Check sheet for the modelled part. Datum: model origin and axes. Units: mm. Round coordinates to 2 decimals unless told otherwise and drop trailing zeros. Order: outer loops, then holes, each group sorted by start corner. A loop starts at its lowest first (then second) coordinate and runs counter-clockwise, first axis right, second up. Notation, with made-up numbers: M -18.5,89 L 9.5,89 A18 cw 9.5,115 Z; hole C 80,89.5 d10. An arc over 180 degrees is marked long. One line per item, written item: value. Start each with the question number.
(1) Thickness scan on L1, parallel to X at y = 5, z = -61.5; L2, parallel to X at y = 4, z = -65 (1 decimal); L3, parallel to Z at x = 895.35, y = 6. Record the ranges inside material, lowest first.
(2) Cross-section at A-A, the plane z = -52. Enter the section's corners in (x, y) (3 decimals), and give its area (3 significant figures).
(3) Cross-section at C-C, the plane y = 5. Count the separate pieces of the cut face and the enclosed holes in it, and give its area (3 significant figures).
(4) Depth check by flat-ended pin: pin 1 Ø5 at (x, y) = (202.5, 8) entering from -Z. Enter the tip coordinate at first touch or a pass-through.
(5) Cross-section at D-D, the plane x = 307. Enter the section's corners in (y, z) (3 decimals).
(6) Cross-section at B-B, the plane x = 756. Enter the section's corners in (y, z) (3 decimals).
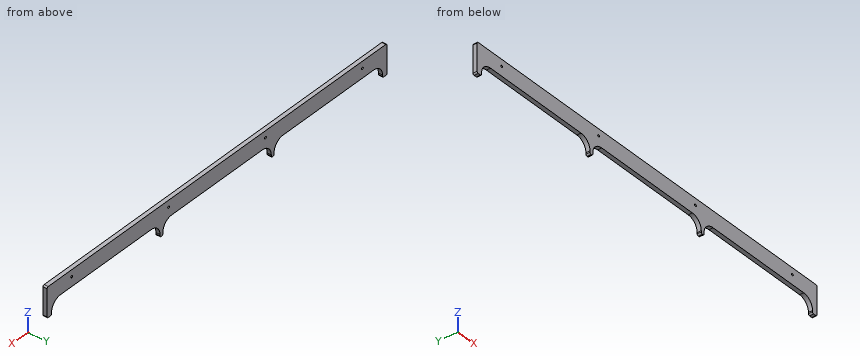
from build123d import *

# Parameters (mm, degrees)
SKETCH1_R           = 2.45745
BOSS_EXTRUDE1_DEPTH = 9.525
FILLET1_R           = 3.175


with BuildPart() as part:
    # Sketch1 → Boss-Extrude1 (new body)
    with BuildSketch(Plane(origin=(0, 0, 0), x_dir=(1, 0, 0), z_dir=(0, 1, 0))):
        with BuildLine():
            Line((0, 0), (965.2, 0))
            Line((965.2, 0), (965.2, 69.85))
            Line((965.2, 69.85), (952.5, 69.85))
            Line((952.5, 69.85), (952.5, 63.5))
            ThreePointArc((952.5, 63.5), (945.060512242, 45.539487758), (927.1, 38.1))
            Line((927.1, 38.1), (669.925, 38.1))
            ThreePointArc((669.925, 38.1), (651.964487758, 45.539487758), (644.525, 63.5))
            Line((644.525, 63.5), (644.525, 69.85))
            Line((644.525, 69.85), (636.5875, 69.85))
            Line((636.5875, 69.85), (636.5875, 63.5))
            ThreePointArc((636.5875, 63.5), (629.148012242, 45.539487758), (611.1875, 38.1))
            Line((611.1875, 38.1), (354.0125, 38.1))
            ThreePointArc((354.0125, 38.1), (336.051987758, 45.539487758), (328.6125, 63.5))
            Line((328.6125, 63.5), (328.6125, 69.85))
            Line((328.6125, 69.85), (320.675, 69.85))
            Line((320.675, 69.85), (320.675, 63.5))
            ThreePointArc((320.675, 63.5), (313.235512242, 45.539487758), (295.275, 38.1))
            Line((295.275, 38.1), (38.1, 38.1))
            ThreePointArc((38.1, 38.1), (20.139487758, 45.539487758), (12.7, 63.5))
            Line((12.7, 63.5), (12.7, 69.85))
            Line((12.7, 69.85), (0, 69.85))
            Line((0, 69.85), (0, 0))
        make_face()
        with Locations(Location((69.85, 15.875, 0), (0, 0, 90))):
            Circle(SKETCH1_R, mode=Mode.SUBTRACT)
        with Locations(Location((345.01582, 15.875, 0), (0, 0, 90))):
            Circle(SKETCH1_R, mode=Mode.SUBTRACT)
        with Locations(Location((895.35, 15.875, 0), (0, 0, 90))):
            Circle(SKETCH1_R, mode=Mode.SUBTRACT)
        with Locations(Location((620.18418, 15.875, 0), (0, 0, 90))):
            Circle(SKETCH1_R, mode=Mode.SUBTRACT)
    extrude(amount=BOSS_EXTRUDE1_DEPTH)

    # Fillet1
    fillet1_edges = [part.edges().sort_by_distance(p)[0] for p in [
        (0, 4.7625, -69.85),
        (12.7, 4.7625, -69.85),
        (320.675, 4.7625, -69.85),
        (328.6125, 4.7625, -69.85),
        (636.5875, 4.7625, -69.85),
        (644.525, 4.7625, -69.85),
        (952.5, 4.7625, -69.85),
        (965.2, 4.7625, -69.85),
        (965.2, 4.7625, 0),
        (0, 4.7625, 0),
    ]]
    fillet(fillet1_edges, radius=FILLET1_R)


solid = part.part
Values found:
1. L1: 0 to 12.78, 320.6 to 328.69, 636.51 to 644.6, 952.42 to 965.2
1. L2: 0 to 12.7, 320.7 to 328.6, 636.6 to 644.5, 952.5 to 965.2
1. L3: -38.1 to -18.33, -13.42 to 0
2. outline: M 0,0 L 15.452,0 L 15.452,9.525 L 0,9.525 Z; M 317.923,0 L 331.365,0 L 331.365,9.525 L 317.923,9.525 Z; M 633.835,0 L 647.277,0 L 647.277,9.525 L 633.835,9.525 Z; M 949.748,0 L 965.2,0 L 965.2,9.525 L 949.748,9.525 Z
2. area: 550 mm^2
3. separate pieces: 1
3. enclosed holes: 4
3. area: 38,800 mm^2
4. pin 1: z = -38.1
5. outline: M 0,-40.968 L 9.525,-40.968 L 9.525,0 L 0,0 Z
6. outline: M 0,-38.1 L 9.525,-38.1 L 9.525,0 L 0,0 Z
